Autodesk Inventor part; units mm, degrees
ref_plane "Start Plane" through (0, 0, 0) normal (0, 0, 1) x (1, 0, 0)
ref_plane "End Plane" through (0, 0, 355) normal (0, 0, 1) x (1, 0, 0)
ref_plane "Work Plane11" through (8.0498, -11.9502, 355) normal (0, 0.7071, 0.7071) x (1, 0, 0)
ref_plane "Start Plane" through (0, 0, 0) normal (0, 0, 1) x (1, 0, 0)
ref_plane "End Plane" through (0, 0, 355) normal (0, 0, 1) x (1, 0, 0)
sketch "Sketch" plane through (0, 0, 0) normal (0, 0, 1) x (1, 0, 0)
  line L0 (-5.9502, 0.0498) -> (-5.9502, 25.6498)
  line L1 (-11.9502, 28.0498) -> (-8.3502, 28.0498)
  line L2 (-11.9502, -11.9502) -> (-11.9502, 28.0498)
  line L3 (-11.9502, -11.9502) -> (28.0498, -11.9502)
  line L4 (28.0498, -8.3502) -> (28.0498, -11.9502)
  line L5 (0.0498, -5.9502) -> (25.6498, -5.9502)
  arc A0 (-5.9502, 0.0498) -> (0.0498, -5.9502) centre (0.0498, 0.0498) ccw
  arc A1 (-5.9502, 25.6498) -> (-8.3502, 28.0498) centre (-8.3502, 25.6498) ccw
  arc A2 (28.0498, -8.3502) -> (25.6498, -5.9502) centre (25.6498, -8.3502) ccw
  line L6 (0, 36.6463) -> (0, -20.0496) construction
  line L7 (-20.0496, 0) -> (36.6463, 0) construction
  point P0 (-5.9502, -5.9502)
  point P1 (-5.9502, 28.0498)
  point P2 (28.0498, -5.9502)
  dimension "d4" = 40
  dimension "d6" = 40
  dimension "d8" = 6
  dimension "d10" = 6
  dimension "d17" = 6
  dimension "d18" = 2.4
  dimension "d19" = 11.9502
  dimension "d20" = 11.9502
extrude "Body" add sketch "Sketch" along normal up to surface (355 mm away) from surface at 0
sketch "Sketch3" plane through (0, 0, 0) normal (0, 0, 1) x (1, 0, 0)
  line L0 (0, 0) -> (10, 0)
ref_plane "Work Plane10" through (0, 0, 0) normal (0, -1, 0) x (1, 0, 0)
sketch "Sketch4" plane through (0, 0, 0) normal (0, -1, 0) x (1, 0, 0)
  line L0 (-2, 0) -> (12, 0)
  line L1 (-2, 355) -> (12, 355)
  dimension "d24" = 355
ref_plane "Work Plane11" through (8.0498, -11.9502, 355) normal (0, 0.7071, 0.7071) x (1, 0, 0)
split "Split1" plane through (8.0498, -11.9502, 355) removes the side toward (0, 0.7071, 0.7071)
ref_plane "Work Plane12" through (8.0498, -11.9502, 0) normal (0, 0.7071, -0.7071) x (1, 0, 0)
split "Split2" plane through (8.0498, -11.9502, 0) removes the side toward (0, 0.7071, -0.7071)
equation "\"d4\" = b"
equation "\"d6\" = b"
equation "\"d17\" = R"
equation "\"d18\" = R1"
equation "\"d19\" = ex"
equation "\"d20\" = d19"
equation "\"d11\" = G_L"
equation "\"b\" = 40"
equation "\"ParT\" = 6"
equation "\"R\" = 6"
equation "\"R1\" = 2.4"
equation "\"G_L\" = d24"
equation "\"G_OFFSET_START\" = 0"
equation "\"G_OFFSET_END\" = 0"
equation "\"d22\" = G_OFFSET_END + B_L"
equation "\"B_L\" = 355"
properties part number "BS 4848 - 40x40x6-355" material "Steel, Mild"
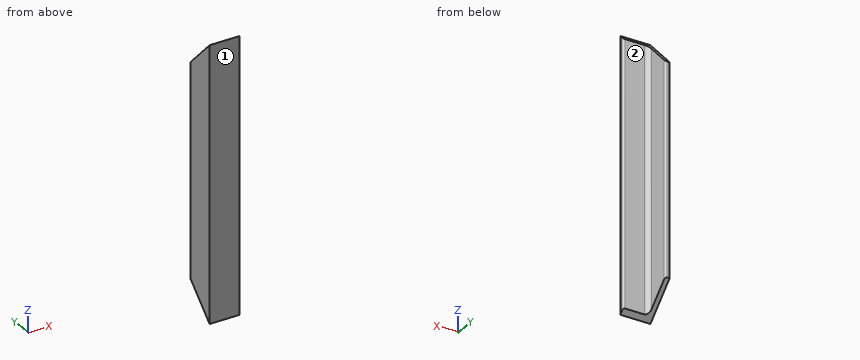
The listing builds one solid part. Answer for the finished solid, in the listing's coordinates (mm). Face numbers are marked on the shaded views. A direction names the side the tool comes from. Coordinates: 2 decimals unless noted, no trailing zeros. Loops run counter-clockwise (first coordinate to the right, second up) from the corner with the lowest first, then second, coordinate; pieces in that order, holes last. Notation, with made-up numbers: (51.5, 62.25) -> (72.5, 62.25) arc R9 cw to (72.5, 67.25) -> close; hole circle Ø3 at (-14, 36.25). An arc over 180 degrees is marked (long way). Write item = value, one per line. Start each with the question number.
1) A cutting plane is placed at C-C (y = 5). Give the vertices of the cut face in (x, z).
2) A tool of negligible diameter and unlimited length cuts with its end or side. For the marked faces 1 and 2, from which of +Z, -Z, +X, -X, +Y, -Y can it reach the whole face along a straight path? Write none if from no direction.
3) A cutting plane is placed at A-A (z = 274). Give the vertices of the cut face in (x, y).
4) Straight lines are drawn through the part: line 1 (X direction, y = 21, z = 210.5); line 2 (X direction, y = -0.5, z = 175). For each, find the intervals that lie inside material, in ascending order. Write a range as from..to.
5) Given pin 1 Ø13 at (y, z) = (11.5, 150.5) entering from +X; pin 2 Ø13 at (x, z) = (17.5, 237.5) entering from +Y; pin 3 Ø10 at (x, y) = (-7.5, 15.5) entering from -Z, each flat-ended and moving along its own axis, determine where each tip first touches the part or whether it passes through.
6) A cutting plane is placed at B-B (x = 10). Give the vertices of the cut face in (y, z), then the cut area to 3 significant figures.
7) A cutting plane is placed at D-D (z = 28). Give the vertices of the cut face in (x, y), then the cut area to 3 significant figures.
Responses:
q1.outline = (-11.95, 16.95) -> (-5.95, 16.95) -> (-5.95, 338.05) -> (-11.95, 338.05) -> close
q2.face_1 = +Z, -Z, +X, -X, -Y
q2.face_2 = +Z, -Z, +X, +Y
q3.outline = (-11.95, -11.95) -> (28.05, -11.95) -> (28.05, -8.35) arc R2.4 ccw to (25.65, -5.95) -> (0.05, -5.95) arc R6 cw to (-5.95, 0.05) -> (-5.95, 25.65) arc R2.4 ccw to (-8.35, 28.05) -> (-11.95, 28.05) -> close
q4.line_1 = -11.95..-5.95
q4.line_2 = -11.95..-5.92
q5.pin_1 = -5.95
q5.pin_2 = -5.95
q5.pin_3 = 22.45
q6.outline = (-11.95, 0) -> (-5.95, 6) -> (-5.95, 349) -> (-11.95, 355) -> close
q6.area = 2,090 mm²
q7.outline = (-11.95, -11.95) -> (28.05, -11.95) -> (28.05, -8.35) arc R2.4 ccw to (25.65, -5.95) -> (0.05, -5.95) arc R6 cw to (-5.95, 0.05) -> (-5.95, 16.05) -> (-11.95, 16.05) -> close
q7.area = 378 mm²
